Check sheet for the modelled part. Datum: model origin and axes. Units: mm. Face numbers are marked on the shaded views. Round coordinates to 2 decimals unless told otherwise and drop trailing zeros. Loops run counter-clockwise (first coordinate to the right, second up) from the corner with the lowest first, then second, coordinate; pieces in that order, holes last. Notation, with made-up numbers: (35.5, 1.5) - (79.5, 1.5) arc R24 cw to (79.5, 19.5) - close; hole circle Ø6 at (40.25, 40.25). An arc over 180 degrees is marked (long way). Put each result on its own line as item: value.
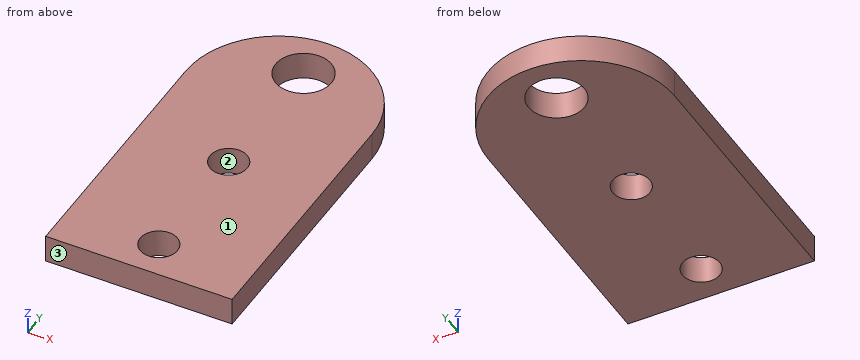
Autodesk Inventor part; units mm, degrees
ref_plane "YZ Plane" through (0, 0, 0) normal (1, 0, 0) x (0, 1, 0)
ref_plane "XZ Plane" through (0, 0, 0) normal (0, 1, 0) x (-1, 0, 0)
ref_plane "XY Plane" through (0, 0, 0) normal (0, 0, 1) x (1, 0, 0)
sketch "Náčrt1" plane through (0, 0, 0) normal (0, 0, 1) x (1, 0, 0)
  line L0 (0, 19) -> (0, 19)
  line L1 (5, 14) -> (5, 0)
  line L2 (0, -19) -> (0, -19)
  line L3 (-5, 0) -> (-5, 14)
  line L4 (-8.4497, 0) -> (8.4497, 0)
  line L5 (0, 27.8426) -> (0, -26.8071)
  arc A0 (0, 19) -> (-5, 14) centre (0, 14) ccw
  arc A1 (5, 14) -> (0, 19) centre (0, 14) ccw
  line L6 (-5, 0) -> (5, 0)
  point P0 (0, 0)
  point P1 (-5, 19)
  point P2 (5, -19)
  point P3 (5, 19)
  point P4 (0, 19)
  dimension "d2" = 5
  dimension "d12" = 14
  dimension "d13" = 10
extrude "Vysunutí1" add sketch "Náčrt1" along normal mid plane 1.5
sketch "Náčrt2" plane through (0, 0, 0.75) normal (0, 0, 1) x (1, 0, 0)
  line L0 (5, 0) -> (5, 14)
  arc A0 (5, 14) -> (-5, 14) centre (0, 14) ccw
  line L1 (-5, 14) -> (-5, 0)
  line L2 (-5, 0) -> (5, 0)
  line L3 (-7, 0) -> (7, 0)
  line L4 (0, 25.3) -> (0, -18.8)
  point P0 (0, 0)
  point P1 (0, -12.5)
  point P2 (0, 16.5)
  dimension "d23" = 2.5
hole "Díra1" at (0, -12.5, 0.75) at (0, 16.5, 0.75) direction (0, 0, -1) diameter 3 end through all
sketch "Náčrt3" plane through (0, 0, 0.75) normal (0, 0, 1) x (1, 0, 0)
  line L0 (-5, 14) -> (-5, 0)
  line L1 (-5, 0) -> (5, 0)
  line L2 (5, 0) -> (5, 14)
  arc A0 (5, 14) -> (-5, 14) centre (0, 14) ccw
  point P0 (0, 0)
  point P1 (0, 2)
  point P2 (0, 9)
  dimension "d14" = 2
  dimension "d15" = 7
hole "Díra2" at (0, 2, 0.75) at (0, 9, 0.75) direction (0, 0, -1) diameter 2 end through all
properties part number "lifter_servo_end" material "Hliník 6061"
Item 1: Thickness scan on line 1 (Y direction, x = 0, z = 0); line 2 (X direction, y = 9, z = 0.3); line 3 (X direction, y = 16.5, z = 0). Record the ranges inside material, lowest first. Write a range as from..to.
Filled sheet:
line 1: 0..1, 3..8, 10..15, 18..19
line 2: -5..-1, 1..5
line 3: -4.33..-1.5, 1.5..4.33
Item 2: Section check D-D on x = 1.25. Enter the section's corners in (y, z).
Filled sheet:
outline: (0, -0.75) - (15.67, -0.75) - (15.67, 0.75) - (0, 0.75) - close; (17.33, -0.75) - (18.84, -0.75) - (18.84, 0.75) - (17.33, 0.75) - close
Item 3: Release check for a two-part mould opening along Y. For the marked faces 1, 2 and 3 record: +Y half, -Y half, draft (parallel to the pull), parting line (faces both ways), or undercut.
Filled sheet:
face 1: draft
face 2: undercut
face 3: -Y half
Item 4: Section check A-A on x = 0. Enter the section's corners in (y, z).
Filled sheet:
outline: (0, -0.75) - (1, -0.75) - (1, 0.75) - (0, 0.75) - close; (3, -0.75) - (8, -0.75) - (8, 0.75) - (3, 0.75) - close; (10, -0.75) - (15, -0.75) - (15, 0.75) - (10, 0.75) - close; (18, -0.75) - (19, -0.75) - (19, 0.75) - (18, 0.75) - close
Item 5: Section check C-C on z = -0.1. Enter the section's corners in (x, y), then the cut area to 3 significant figures.
Filled sheet:
outline: (-5, 0) - (5, 0) - (5, 14) arc R5 ccw to (-5, 14) - close; hole circle Ø3 at (0, 16.5); hole circle Ø2 at (0, 2); hole circle Ø2 at (0, 9)
area: 166 mm²
Item 6: Section check B-B on y = 9. Enter the section's corners in (x, z).
Filled sheet:
outline: (-5, -0.75) - (-1, -0.75) - (-1, 0.75) - (-5, 0.75) - close; (1, -0.75) - (5, -0.75) - (5, 0.75) - (1, 0.75) - close
